Source: three-view drawing plus pictorial views. Frame: mm from the lowest corner of the part. Give positions to 0.01 mm unless a question says otherwise; leave off trailing zeros. Order: outer loops, then holes, each group sorted by start corner. A loop starts at its lowest first (then second) coordinate and runs counter-clockwise, first axis right, second up.
1) Section A-A, the plane x = 5. Return loops of the section in (y, z).
2) First-contact query: P1, Ø3.5, axis at x = 5, z = 15, coming from the +Y side (3 decimals). Flat tip, straight axial feed; report the tip coordinate or a pass-through.
3) Material intervals for line 1 (X direction, y = 7.25, z = 15); line 2 (Z direction, x = 5, y = 7.25), sorted ascending.
4) Section B-B, the plane z = 15. Return loops of the section in (x, y), plus the area to 3 significant figures.
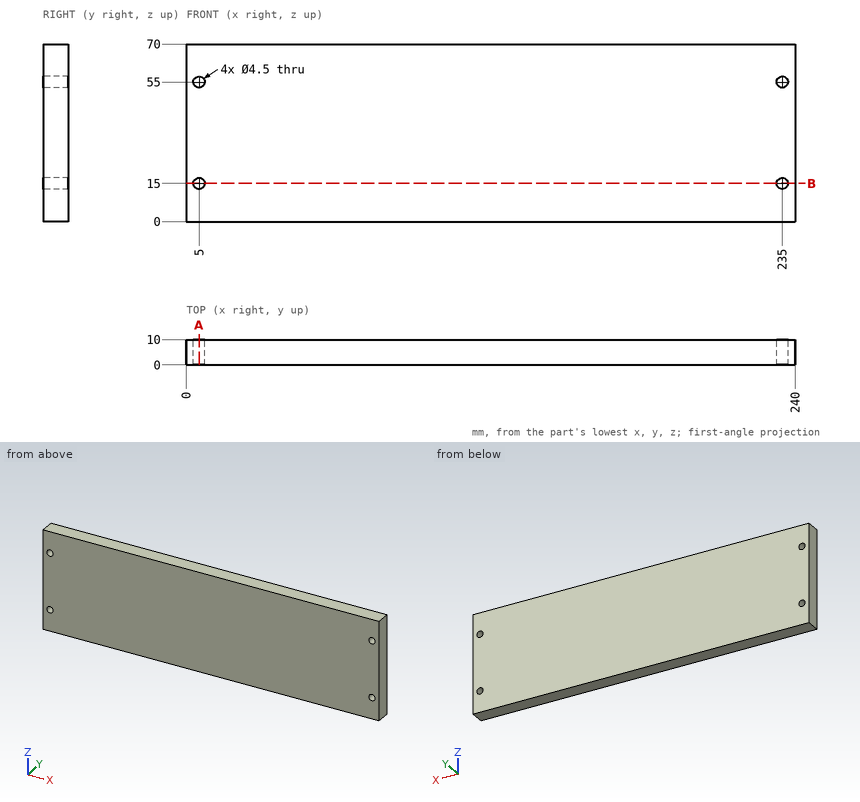
From the geometry:
1. outline: (0, 0) - (10, 0) - (10, 12.75) - (0, 12.75) - close; (0, 17.25) - (10, 17.25) - (10, 52.75) - (0, 52.75) - close; (0, 57.25) - (10, 57.25) - (10, 70) - (0, 70) - close
2. P1: passes through
3. line 1: x = 0 to 2.75, 7.25 to 232.75, 237.25 to 240
3. line 2: z = 0 to 12.75, 17.25 to 52.75, 57.25 to 70
4. outline: (0, 0) - (2.75, 0) - (2.75, 10) - (0, 10) - close; (7.25, 0) - (232.75, 0) - (232.75, 10) - (7.25, 10) - close; (237.25, 0) - (240, 0) - (240, 10) - (237.25, 10) - close
4. area: 2,310 mm2
